from build123d import *

# Parameters (mm, degrees)
SKETCH3_W           = 180
SKETCH3_H           = 70
BOSS_EXTRUDE1_DEPTH = 3
SKETCH5_W           = 3
SKETCH5_H           = 5
CUT_EXTRUDE2_DEPTH  = 3
SKETCH4_W           = 35
SKETCH4_H           = 3
SKETCH4_W_2         = 40
CUT_EXTRUDE3_DEPTH  = 10


with BuildPart() as part:
    # Sketch3 → Boss-Extrude1 (new body)
    with BuildSketch(Plane.XY):
        Rectangle(SKETCH3_W, SKETCH3_H)
    extrude(amount=BOSS_EXTRUDE1_DEPTH)

    # Sketch5 → Cut-Extrude2 (cut)
    with BuildSketch(Plane.XY.offset(3)):
        with Locations((-88.5, 2.5)):
            Rectangle(SKETCH5_W, SKETCH5_H)
        with Locations((-88.5, -2.5)):
            Rectangle(SKETCH5_W, SKETCH5_H)
        with Locations((88.5, 2.5)):
            Rectangle(SKETCH5_W, SKETCH5_H)
        with Locations((88.5, -2.5)):
            Rectangle(SKETCH5_W, SKETCH5_H)
    extrude(amount=-CUT_EXTRUDE2_DEPTH, mode=Mode.SUBTRACT)

    # Sketch4 → Cut-Extrude3 (cut)
    with BuildSketch(Plane.XY.offset(3)):
        with Locations((-72.5, 33.5)):
            Rectangle(SKETCH4_W, SKETCH4_H)
        with Locations((-25, 33.5)):
            Rectangle(SKETCH4_W_2, SKETCH4_H)
        with Locations((25, 33.5)):
            Rectangle(SKETCH4_W_2, SKETCH4_H)
        with Locations((72.5, 33.5)):
            Rectangle(SKETCH4_W, SKETCH4_H)
        with Locations((72.5, -33.5)):
            Rectangle(SKETCH4_W, SKETCH4_H)
        with Locations((25, -33.5)):
            Rectangle(SKETCH4_W_2, SKETCH4_H)
        with Locations((-25, -33.5)):
            Rectangle(SKETCH4_W_2, SKETCH4_H)
        with Locations((-72.5, -33.5)):
            Rectangle(SKETCH4_W, SKETCH4_H)
    extrude(amount=-CUT_EXTRUDE3_DEPTH, mode=Mode.SUBTRACT)


solid = part.part
For this review, take the finished solid that the model builds, in its own axes (mm). A direction names the side the tool comes from. Round coordinates to 2 decimals unless told otherwise and drop trailing zeros. Loops run counter-clockwise (first coordinate to the right, second up) from the corner with the lowest first, then second, coordinate; pieces in that order, holes last. Notation, with made-up numbers: (-32.5, -8) - (0.5, -8) arc R17 ccw to (0.5, 24) - close; hole circle Ø8 at (53.5, -19). An arc over 180 degrees is marked (long way). One line per question, with ' | ' between items.
Q1. The part is to be moulded in two halves that separate along Y. For faces 1 (the flat face through (88, -5, 2)), 2 (the flat face through (-50, -35, 1)), 3 (the flat face through (90, 18, 1)), say which applies: released by +Y, released by -Y, zero draft, split by the parting line, or undercut.
Taken from the geometry:
face 1: undercut | face 2: released by -Y | face 3: zero draft
Q2. Take a section at A-A (x = -16.5). Give the boundary of the cut face in (y, z).
Taken from the geometry:
outline: (-32, 0) - (32, 0) - (32, 3) - (-32, 3) - close
Q3. Take a section at B-B (y = -2). Give the boundary of the cut face in (x, z), and give its area (3 significant figures).
Taken from the geometry:
outline: (-87, 0) - (87, 0) - (87, 3) - (-87, 3) - close | area: 522 mm²
Q4. For pin 1 (0.9 mm diameter, centred on x = 79.5, z = 1, fed in from -Y); pin 2 (1.5 mm diameter, centred on y = 33.5, z = 2, fed in from -X); pin 3 (0.9 mm diameter, centred on x = -80, z = 1, fed in from +Y), all flat-tipped, find the tip position at first contact; note any pin that passes through.
Taken from the geometry:
pin 1: stops at y = -32 | pin 2: stops at x = -55 | pin 3: stops at y = 32
Q5. Tool access review of faces 4 (the flat face through (55, -34, 2)), 5 (the flat face through (-45, 33, 2)), 6 (the flat face through (-55, 33, 2)): name each direction out of +Z, -Z, +X, -X, +Y, -Y from which nothing blocks a thin tool from reaching the whole face with its end or side.
Taken from the geometry:
face 4: +Z, -Z, +X, -Y | face 5: +Z, -Z, +Y | face 6: +Z, -Z, -X, +Y
Q6. For line 1 along Y through (x, z) = (-62.5, 1.2); line 2 along X through (y, z) = (-2, 2.45), list the stretches that pass through material, from the lowest coordinate up. Write a range as [from, to].
Taken from the geometry:
line 1: y = [-32, 32] | line 2: x = [-87, 87]
